The drawing under review shows one solid part. Ordinate dimensions are in mm from its lowest x, y, z. A direction names the side the tool comes from. Round coordinates to 2 decimals unless told otherwise and drop trailing zeros. Loops run counter-clockwise (first coordinate to the right, second up) from the corner with the lowest first, then second, coordinate; pieces in that order, holes last. Notation, with made-up numbers: M 9.25,34.5 L 54.25,34.5 A12 cw 54.25,41.5 Z; hole C 52,86.25 d4. An arc over 180 degrees is marked long. Use a Markdown table: item, result.
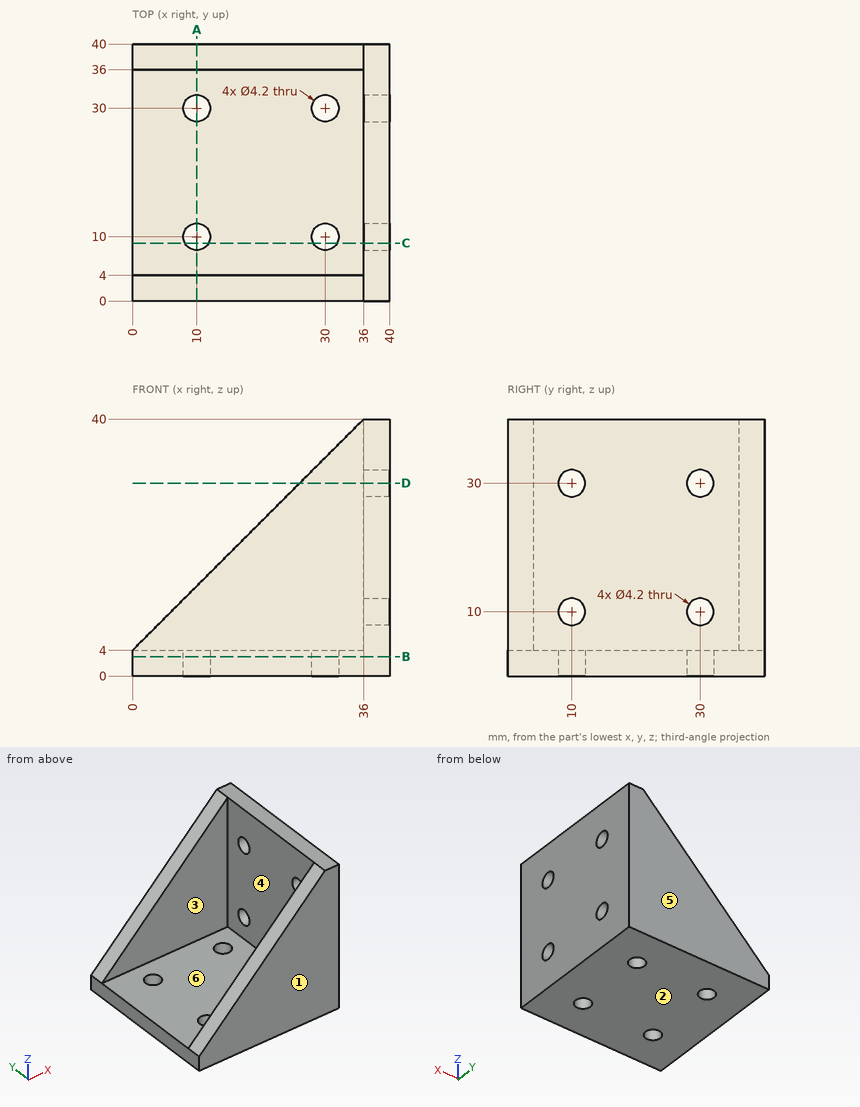
1. Insertion check: pin 1 (16 mm diameter, centred on x = 17, y = 19, fed in from +Z); pin 2 (3.5 mm diameter, centred on x = 30, y = 30, fed in from -Z); pin 3 (5 mm diameter, centred on y = 30, z = 30, fed in from -X). Each pin has a flat end and moves straight along its axis. Give the tip position at first contact, or say it passes through.
Check values:
| item | result |
|---|---|
| pin 1 | stops at z = 4 |
| pin 2 | passes through |
| pin 3 | stops at x = 36 |
2. Machinability: for the marked faces 5 and 6, which of the approach directions +Z, -Z, +X, -X, +Y, -Y give a long, thin tool a straight path to every point of the face, cutting with its end or side? Answer none if there is none.
Check values:
| item | result |
|---|---|
| face 5 | +Z, -Z, +X, -X, +Y |
| face 6 | +Z, -X |
3. Take a section at D-D on z = 30. Give the boundary of the cut face in (x, y).
Check values:
| item | result |
|---|---|
| outline | M 26,0 L 40,0 L 40,7.9 L 36,7.9 L 36,4 L 26,4 Z; M 26,36 L 36,36 L 36,32.1 L 40,32.1 L 40,40 L 26,40 Z; M 36,12.1 L 40,12.1 L 40,27.9 L 36,27.9 Z |
4. The part is to be moulded in two halves that separate along Y. For the marked faces 1, 2, 3 and 4, say which applies: pulls with the +Y half, pulls with the -Y half, needs draft (parallel to the pull), parting line crosses it, or undercut.
Check values:
| item | result |
|---|---|
| face 1 | pulls with the -Y half |
| face 2 | needs draft |
| face 3 | undercut |
| face 4 | undercut |
5. Wall thickness on line 1 along Y through (x, z) = (10, 3.05); line 2 along Y through (x, z) = (33.5, 29.5); line 3 along Z through (x, y) = (25, 25.5): over which ranges is each line inside the solid? List them lowest first. Write a range as from..to.
Check values:
| item | result |
|---|---|
| line 1 | y = 0..7.9, 12.1..27.9, 32.1..40 |
| line 2 | y = 0..4, 36..40 |
| line 3 | z = 0..4 |
6. Take a section at A-A on x = 10. Give the boundary of the cut face in (y, z).
Check values:
| item | result |
|---|---|
| outline | M 0,0 L 7.9,0 L 7.9,4 L 4,4 L 4,14 L 0,14 Z; M 12.1,0 L 27.9,0 L 27.9,4 L 12.1,4 Z; M 32.1,0 L 40,0 L 40,14 L 36,14 L 36,4 L 32.1,4 Z |
7. Take a section at B-B on z = 3. Give the boundary of the cut face in (x, y), and give its area (3 significant figures).
Check values:
| item | result |
|---|---|
| outline | M 0,0 L 40,0 L 40,40 L 0,40 Z; hole C 10,10 d4.2; hole C 10,30 d4.2; hole C 30,10 d4.2; hole C 30,30 d4.2 |
| area | 1,540 mm² |
8. Take a section at C-C on y = 9. Give the boundary of the cut face in (x, z).
Check values:
| item | result |
|---|---|
| outline | M 0,0 L 8.15,0 L 8.15,4 L 0,4 Z; M 11.85,0 L 28.15,0 L 28.15,4 L 11.85,4 Z; M 31.85,0 L 40,0 L 40,8.15 L 36,8.15 L 36,4 L 31.85,4 Z; M 36,11.85 L 40,11.85 L 40,28.15 L 36,28.15 Z; M 36,31.85 L 40,31.85 L 40,40 L 36,40 Z |
